from build123d import *
from build123d.topology import SkipClean

# Parameters (mm, degrees)
SKETCH1_W           = 88.9
SKETCH1_H           = 28.575
SKETCH1_R           = 2.25
BOSS_EXTRUDE1_DEPTH = 6.35
SKETCH2_W           = 24.575
SKETCH2_H           = 28.575
SKETCH2_R           = 2.25
SKETCH2_W_2         = 6.35
SKETCH2_H_2         = 6.35
SKETCH2_W_3         = 7.175
BOSS_EXTRUDE2_DEPTH = 6.35
SKETCH2_4_W         = 6.35
SKETCH2_4_H         = 28.575
BOSS_EXTRUDE3_DEPTH = 38.1
BOSS_EXTRUDE4_DEPTH = 6.35
CUT_EXTRUDE1_DEPTH  = 97.028
BOSS_EXTRUDE5_START = -6.35
BOSS_EXTRUDE5_DEPTH = 6.35
FILLET1_R           = 3.175


with BuildPart() as part:
    # Sketch1 → Boss-Extrude1 (new body)
    with BuildSketch(Plane.XY):
        Rectangle(SKETCH1_W, SKETCH1_H)
        with Locations((-38.066912716, -1.5875)):
            Circle(SKETCH1_R, mode=Mode.SUBTRACT)
        with Locations((0.033087284, -1.5875)):
            Circle(SKETCH1_R, mode=Mode.SUBTRACT)
        with Locations((38.133087284, -1.5875)):
            Circle(SKETCH1_R, mode=Mode.SUBTRACT)
    extrude(amount=BOSS_EXTRUDE1_DEPTH)

    # Sketch2 → Boss-Extrude2 (add)
    # profile 1 of 10: a face of its own
    with BuildSketch(Plane(origin=(0, 14.2875, 0), x_dir=(1, 0, 0), z_dir=(0, 1, 0))):
        with Locations((-32.1625, 14.2875)):
            Rectangle(SKETCH2_W, SKETCH2_H)
        with Locations(Location((-38.1, 15.875, 0), (0, 0, 180))):
            Circle(SKETCH2_R, mode=Mode.SUBTRACT)
    # profile 2 of 10: a face of its own
    with BuildSketch(Plane(origin=(0, 14.2875, 0), x_dir=(1, 0, 0), z_dir=(0, 1, 0))):
        with Locations((-16.7, 14.2875)):
            Rectangle(SKETCH2_W_2, SKETCH2_H)
    # profile 3 of 10: a face of its own
    with BuildSketch(Plane(origin=(0, 14.2875, 0), x_dir=(1, 0, 0), z_dir=(0, 1, 0))):
        with Locations((-32.1625, -3.175)):
            Rectangle(SKETCH2_W, SKETCH2_H_2)
    # profile 4 of 10: a face of its own
    with BuildSketch(Plane(origin=(0, 14.2875, 0), x_dir=(1, 0, 0), z_dir=(0, 1, 0))):
        with Locations((-16.7, -3.175)):
            Rectangle(SKETCH2_W_2, SKETCH2_H_2)
    # profile 5 of 10: a face of its own
    with BuildSketch(Plane(origin=(0, 14.2875, 0), x_dir=(1, 0, 0), z_dir=(0, 1, 0))):
        Polygon((-13.525, 28.575), (-13.525, 0), (30.925, 0), (30.925, 28.575), (21.4, 28.575), (-4, 28.575), align=None)
        with Locations(Location((0, 15.875, 0), (0, 0, 180))):
            Circle(SKETCH2_R, mode=Mode.SUBTRACT)
    # profile 6 of 10: a face of its own
    with BuildSketch(Plane(origin=(0, 14.2875, 0), x_dir=(1, 0, 0), z_dir=(0, 1, 0))):
        Polygon((-13.525, 0), (-13.525, -6.35), (-4, -6.35), (21.4, -6.35), (30.925, -6.35), (30.925, 0), align=None)
    # profile 7 of 10: a face of its own
    with BuildSketch(Plane(origin=(0, 14.2875, 0), x_dir=(1, 0, 0), z_dir=(0, 1, 0))):
        with Locations((34.1, 14.2875)):
            Rectangle(SKETCH2_W_2, SKETCH2_H)
    # profile 8 of 10: a face of its own
    with BuildSketch(Plane(origin=(0, 14.2875, 0), x_dir=(1, 0, 0), z_dir=(0, 1, 0))):
        with Locations((40.8625, 14.2875)):
            Rectangle(SKETCH2_W_3, SKETCH2_H)
    # profile 9 of 10: a face of its own
    with BuildSketch(Plane(origin=(0, 14.2875, 0), x_dir=(1, 0, 0), z_dir=(0, 1, 0))):
        with Locations((40.8625, -3.175)):
            Rectangle(SKETCH2_W_3, SKETCH2_H_2)
    # profile 10 of 10: a face of its own
    with BuildSketch(Plane(origin=(0, 14.2875, 0), x_dir=(1, 0, 0), z_dir=(0, 1, 0))):
        with Locations((34.1, -3.175)):
            Rectangle(SKETCH2_W_2, SKETCH2_H_2)
    extrude(amount=BOSS_EXTRUDE2_DEPTH)

    # Sketch2<4> → Boss-Extrude3 (add)
    with BuildSketch(Plane(origin=(0, 14.2875, 0), x_dir=(1, 0, 0), z_dir=(0, 1, 0))):
        with Locations((-16.7, 14.2875)):
            Rectangle(SKETCH2_4_W, SKETCH2_4_H)
        with Locations((34.1, 14.2875)):
            Rectangle(SKETCH2_4_W, SKETCH2_4_H)
    extrude(amount=BOSS_EXTRUDE3_DEPTH)

    # Sketch3 → Boss-Extrude4 (add)
    with BuildSketch(Plane.ZY.offset(19.875)):
        with BuildLine():
            ThreePointArc((0, 20.6375), (5.69066224, 21.969154609), (10.199570624, 25.687579802))
            ThreePointArc((10.199570624, 25.687579802), (12.150928324, 29.359383395), (12.825, 33.4625))
            ThreePointArc((12.825, 33.4625), (9.068644469, 42.531144469), (0, 46.2875))
            Line((0, 46.2875), (0, 41.4625))
            ThreePointArc((0, 41.4625), (5.656854249, 39.119354249), (8, 33.4625))
            ThreePointArc((8, 33.4625), (5.656854249, 27.805645751), (0, 25.4625))
            Line((0, 25.4625), (0, 20.6375))
        make_face()
        with BuildLine():
            ThreePointArc((-9.582018268, 41.986909124), (-11.700559218, 28.21106791), (0, 20.6375))
            Line((0, 20.6375), (0, 25.4625))
            ThreePointArc((0, 25.4625), (-8, 33.4625), (0, 41.4625))
            Line((0, 41.4625), (0, 46.2875))
            ThreePointArc((0, 46.2875), (-5.25143209, 45.163059218), (-9.582018268, 41.986909124))
        make_face()
        with BuildLine():
            Line((0, 20.6375), (6.35, 20.6375))
            Line((6.35, 20.6375), (10.199570624, 25.687579802))
            ThreePointArc((10.199570624, 25.687579802), (5.69066224, 21.969154609), (0, 20.6375))
        make_face()
    extrude(amount=-BOSS_EXTRUDE4_DEPTH)

    # Sketch3<4> → Cut-Extrude1 (cut)
    with SkipClean():  # the faces are left unmerged after this step: merging them gives an invalid solid
        with BuildSketch(Plane.ZY.offset(19.875)):
            with BuildLine():
                Line((-28.575, 20.6375), (-9.582018268, 41.986909124))
                ThreePointArc((-9.582018268, 41.986909124), (-5.25143209, 45.163059218), (0, 46.2875))
                Line((0, 46.2875), (0, 52.3875))
                Line((0, 52.3875), (-28.575, 52.3875))
                Line((-28.575, 52.3875), (-28.575, 20.6375))
            make_face()
            with BuildLine():
                Line((0, 41.4625), (0, 25.4625))
                ThreePointArc((0, 25.4625), (5.656854249, 27.805645751), (8, 33.4625))
                ThreePointArc((8, 33.4625), (5.656854249, 39.119354249), (0, 41.4625))
            make_face()
            with BuildLine():
                ThreePointArc((0, 41.4625), (-8, 33.4625), (0, 25.4625))
                Line((0, 25.4625), (0, 41.4625))
            make_face()
        extrude(amount=-CUT_EXTRUDE1_DEPTH, mode=Mode.SUBTRACT)

    # Sketch4 → Boss-Extrude5 (add)
    with SkipClean():  # the faces are left unmerged after this step: merging them gives an invalid solid
        with BuildSketch(Plane(origin=(37.275, 0, 0), x_dir=(0, 0, -1), z_dir=(1, 0, 0)).offset(BOSS_EXTRUDE5_START)):
            with BuildLine():
                Line((0, 46.2875), (0, 41.4625))
                ThreePointArc((0, 41.4625), (8, 33.4625), (0, 25.4625))
                Line((0, 25.4625), (0, 20.6375))
                Line((0, 20.6375), (28.575, 20.6375))
                Line((28.575, 20.6375), (9.582018268, 41.986909124))
                ThreePointArc((9.582018268, 41.986909124), (5.25143209, 45.163059218), (0, 46.2875))
            make_face()
            with BuildLine():
                Line((-6.35, 20.6375), (0, 20.6375))
                Line((0, 20.6375), (0, 25.4625))
                ThreePointArc((0, 25.4625), (-8, 33.4625), (0, 41.4625))
                Line((0, 41.4625), (0, 46.2875))
                ThreePointArc((0, 46.2875), (-11.493345391, 39.15316224), (-10.199570624, 25.687579802))
                Line((-10.199570624, 25.687579802), (-6.35, 20.6375))
            make_face()
        extrude(amount=BOSS_EXTRUDE5_DEPTH)

    # Fillet1
    fillet1_edges = [part.edges().sort_by_distance(p)[0] for p in [
        (-13.525, 20.6375, -11.1125),
        (-19.875, 20.6375, -11.1125),
        (30.925, 20.6375, -14.2875),
        (37.275, 20.6375, -14.2875),
    ]]
    fillet(fillet1_edges, radius=FILLET1_R)


solid = part.part
Source: CAD feature listing. Evaluate the final solid. Frame: model axes, mm. A direction names the side the tool comes from. Round coordinates to 2 decimals unless told otherwise and drop trailing zeros. Loops run counter-clockwise (first coordinate to the right, second up) from the corner with the lowest first, then second, coordinate; pieces in that order, holes last.
Q1. Access query for faces 1 (the face through (42, 20.638, -11)), 2 (the face through (-34, 20.638, -11)), 3 (the face through (-12.57, 21.54, -10.16)). Directions: +Z, -Z, +X, -X, +Y, -Y. A direction counts if a zero-diameter tool reaches every point of the face in a straight line with its end or side. Return the directions, or none.
Q2. Section A-A, the plane z = 3. State how many separate pieces and enclosed holes the cut face has, plus the area to 3 significant figures.
Q3. Mould query, pull axis Z, two halves, no side actions, for faces 4 (the face through (-1, 3, 6.35)), 5 (the face through (-1, 17, -28.575)), 6 (the face through (-35.852, 17.418, -15.776)). Classes: pulls with the +Z half, pulls with the -Z half, needs draft (parallel to the pull), parting line crosses it, or undercut.
Q4. First-contact query: P1, Ø13, axis at y = 33.46, z = 0, coming from the +X side; P2, Ø23, axis at x = -4, z = -13.5, coming from the -Y side; P3, Ø2, axis at y = 21.5, z = -5.5, coming from the -X side; P4, Ø14.5, axis at x = 18.5, y = 3, coming from the -Z side. Flat tips, straight axial feed; report the tip coordinate or a pass-through.
Q5. Section B-B, the plane y = 37. Return loops of the section in (x, z) (1 decimal).
Q6. Ray query, line 1 (X direction, y = 25, z = -17) (3 decimals); line 2 (Z direction, x = -38.1, y = 18.25) (3 decimals); line 3 (Y direction, x = -26.5, z = -1). Return the intervals inside material, ascending.
Solutions:
1. face 1: +Z, -Z, +X, +Y
1. face 2: +Z, -Z, -X, +Y
1. face 3: +Z, -Z, +Y
2. separate pieces: 3
2. enclosed holes: 3
2. area: 3,200 mm2
3. face 4: pulls with the +Z half
3. face 5: pulls with the -Z half
3. face 6: undercut
4. P1: passes through
4. P2: stops at y = 14.29
4. P3: stops at x = -44.45
4. P4: stops at z = 0
5. outline: (-19.9, -14) - (-13.5, -14) - (-13.5, -7.2) - (-19.9, -7.2) - close; (-19.9, 7.2) - (-13.5, 7.2) - (-13.5, 12.3) - (-19.9, 12.3) - close; (30.9, -14) - (37.3, -14) - (37.3, -7.2) - (30.9, -7.2) - close; (30.9, 7.2) - (37.3, 7.2) - (37.3, 12.3) - (30.9, 12.3) - close
6. line 1: x = -19.875 to -13.525, 30.925 to 37.275
6. line 2: z = -28.575 to -18.125, -13.625 to 6.35
6. line 3: y = 14.29 to 20.64
